from build123d import *

# Parameters (mm, degrees)
DODANIE_WYCI_GNI_CIE1_DEPTH                          = 8
WYTNIJ_WYCI_GNI_CIE1_DEPTH                           = 8
WYTNIJ_WYCI_GNI_CIE2_DEPTH                           = 42.097445176
WYTNIJ_WYCI_GNI_CIE2_DEPTH_BACK                      = 42.097445176
POG_BIENIE_STO_KOWE_POD_M3_WKR_T_DO_CZ_C_D           = 3.4
POG_BIENIE_STO_KOWE_POD_M3_WKR_T_DO_CZ_C_CSINK_D     = 6.3
POG_BIENIE_STO_KOWE_POD_M3_WKR_T_DO_CZ_C_CSINK_ANGLE = 90
OTWORY_USTALAJ_CE_5_0MM1_D                           = 5.2
SZKIC8_R                                             = 3.25
WYTNIJ_WYCI_GNI_CIE3_DEPTH                           = 10
ZAOKR_GLENIE1_R                                      = 1


with BuildPart() as part:
    # Szkic1 → Dodanie-wyciągnięcie1 (new, symmetric)
    with BuildSketch(Plane.XY):
        Polygon((0, 0), (35, 0), (31.794871795, -20), (0, -20), align=None)
    dodanie_wyci_gni_cie1 = extrude(amount=DODANIE_WYCI_GNI_CIE1_DEPTH, both=True)

    # Lustro1: Dodanie-wyciągnięcie1 across plane
    add(dodanie_wyci_gni_cie1.mirror(Plane(origin=(0, -20, 8), x_dir=(0, 0, 1), z_dir=(1, 0, 0))))

    # Szkic2 → Wytnij-wyciągnięcie1 (cut)
    with BuildSketch(Plane.XY.offset(8)):
        with BuildLine():
            Line((-13, -20), (13, -20))
            ThreePointArc((13, -20), (0, -7), (-13, -20))
        make_face()
    extrude(amount=-WYTNIJ_WYCI_GNI_CIE1_DEPTH, mode=Mode.SUBTRACT)

    # Szkic3 → Wytnij-wyciągnięcie2 (cut, two sides: drawn at the far end of the back side and taken through both)
    with BuildSketch(Plane.XY.offset(-WYTNIJ_WYCI_GNI_CIE2_DEPTH_BACK)):
        with BuildLine():
            ThreePointArc((9, -20), (0, -11), (-9, -20))
            Line((-9, -20), (9, -20))
        make_face()
    extrude(amount=WYTNIJ_WYCI_GNI_CIE2_DEPTH + WYTNIJ_WYCI_GNI_CIE2_DEPTH_BACK, mode=Mode.SUBTRACT)

    # Pogłębienie stożkowe pod M3 wkręt do części metalowych z łbem soczewkowym1 (through all)
    with Locations(Plane(origin=(0, -20, 0), x_dir=(-1, 0, 0), z_dir=(0, -1, 0))):
        with Locations((-25, 0), (25, 0)):
            CounterSinkHole(POG_BIENIE_STO_KOWE_POD_M3_WKR_T_DO_CZ_C_D / 2, POG_BIENIE_STO_KOWE_POD_M3_WKR_T_DO_CZ_C_CSINK_D / 2, counter_sink_angle=POG_BIENIE_STO_KOWE_POD_M3_WKR_T_DO_CZ_C_CSINK_ANGLE)

    # Otwory ustalające Ø5.0mm1 (through all)
    with Locations(Plane(origin=(0, -20, 0), x_dir=(-1, 0, 0), z_dir=(0, -1, 0))):
        with Locations((-17.5, 0), (17.5, 0)):
            Hole(OTWORY_USTALAJ_CE_5_0MM1_D / 2)

    # Szkic8 → Wytnij-wyciągnięcie3 (cut)
    with BuildSketch(Plane(origin=(0, -20, 0), x_dir=(-1, 0, 0), z_dir=(0, -1, 0))):
        with Locations(Location((17.5, 0, 0), (0, 0, 180))):
            Circle(SZKIC8_R)
        with Locations(Location((-17.5, 0, 0), (0, 0, 180))):
            Circle(SZKIC8_R)
    extrude(amount=-WYTNIJ_WYCI_GNI_CIE3_DEPTH, mode=Mode.SUBTRACT)

    # Zaokrąglenie1
    zaokr_glenie1_edges = [part.edges().sort_by_distance(p)[0] for p in [
        (33.397435897, -10, 8),
        (-33.397435897, -10, 8),
        (-33.397435897, -10, -8),
        (0, -11, 0),
        (0, -11, -8),
        (33.397435897, -10, -8),
    ]]
    fillet(zaokr_glenie1_edges, radius=ZAOKR_GLENIE1_R)


solid = part.part
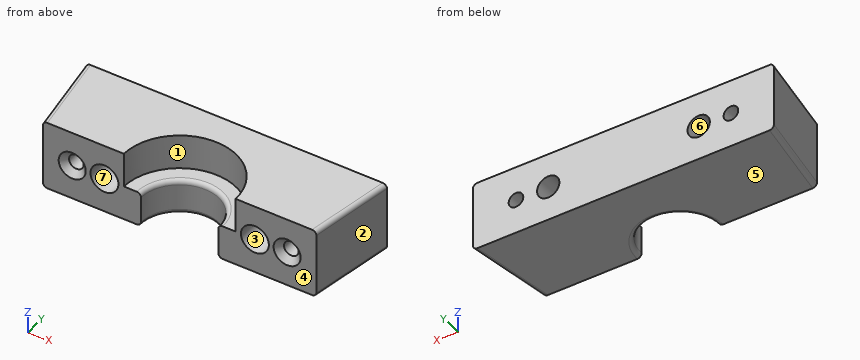
Check sheet for the modelled part. Datum: model origin and axes. Units: mm. Face numbers are marked on the shaded views. A direction names the side the tool comes from. Coordinates: 2 decimals unless noted, no trailing zeros. Write each loop counter-clockwise with the first axis right and the second up, starting at its lowest first coordinate (ties: lowest second). Pieces come first, ordered by that corner, then holes.
Item 1: Cross-section at B-B on z = 4.75. Record the boundary of the cut face in (x, y).
Numbers:
outline: (-35, 0) - (-31.79, -20) - (-13, -20) arc R13 cw to (13, -20) - (31.79, -20) - (35, 0) - close
Item 2: Access from +Z, -Z, +X, -X, +Y, -Y to the whole of each face (thin tool, end or side, straight path). Record for the marked faces 1, 2 and 3.
Numbers:
face 1: +Z, -Y
face 2: +Z, -Z, +X, -Y
face 3: -Y
Item 3: Cross-section at D-D on y = -17.25. Count the separate pieces of the cut face and the enclosed holes in it, then the cut area to 3 significant figures.
Numbers:
separate pieces: 2
enclosed holes: 4
area: 605 mm2
Item 4: Mould release check, pull along Z, two halves, no side actions. Record for the marked faces 4, 5, 6 and 7: released by +Z, released by -Z, zero draft, split by the parting line, or undercut.
Numbers:
face 4: zero draft
face 5: released by -Z
face 6: undercut
face 7: undercut
Item 5: Cross-section at A-A on x = -17.5. Record the boundary of the cut face in (y, z), then the cut area to 3 significant figures.
Numbers:
outline: (-20, -8) - (0, -8) - (0, -2.6) - (-10, -2.6) - (-10, -3.25) - (-20, -3.25) - close; (-20, 3.25) - (-10, 3.25) - (-10, 2.6) - (0, 2.6) - (0, 8) - (-20, 8) - close
area: 203 mm2
Item 6: Scan lines: probe 1 along Z at (x, y) = (-17.5, -4.25); probe 2 along Z at (x, y) = (25, -11.25); probe 3 along Y at (x, z) = (0, -2.5). Record each from-to range of solid material in increasing order.
Numbers:
probe 1: z = -8 to -2.6, 2.6 to 8
probe 2: z = -8 to -1.7, 1.7 to 8
probe 3: y = -11 to 0
Item 7: Cross-section at C-C on x = 0. Record the boundary of the cut face in (y, z).
Numbers:
outline: (-11, -7) arc R1 ccw to (-10, -8) - (0, -8) - (0, 8) - (-7, 8) - (-7, 0) - (-10, 0) arc R1 ccw to (-11, -1) - close
Item 8: Depth check by flat-ended pin: pin 1 Ø6 at (x, z) = (17.5, 0) entering from -Y; pin 2 Ø1.5 at (y, z) = (-2.5, -1.5) entering from +X. Enter the tip coordinate at first touch or a pass-through.
Numbers:
pin 1: stops at y = -10
pin 2: stops at x = 34.72
